Design review of the part shown in the three views and the two pictorial views. Dimensions are in mm from the part's minimum x, y and z. A direction names the side the tool comes from. Round coordinates to 2 decimals unless told otherwise and drop trailing zeros. Order: outer loops, then holes, each group sorted by start corner. A loop starts at its lowest first (then second) coordinate and runs counter-clockwise, first axis right, second up.
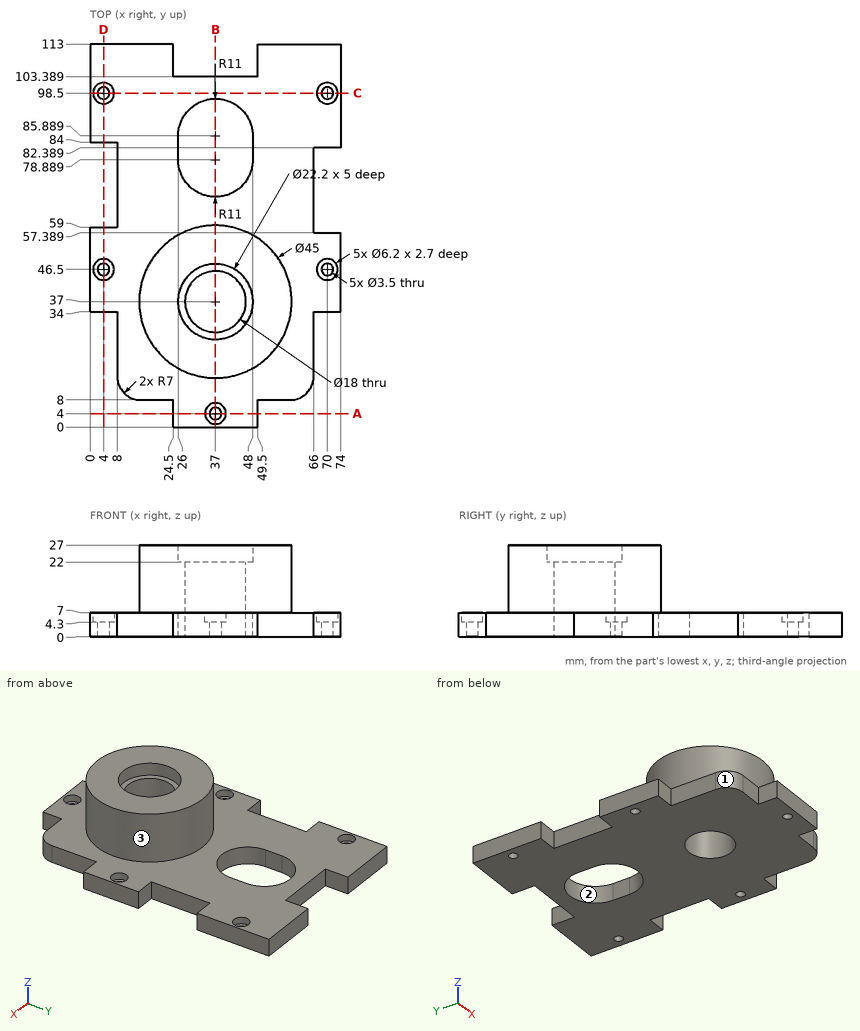
(1) For the marked faces 1, 2 and 3, list the 3-axis set-ups (+Z, -Z, +X, -X, +Y, -Y) from which the entire face can be reached by the end or side of a thin tool; tool diameter is ignored.
Data:
face 1: +Z, -Z, -X, -Y
face 2: +Z, -Z
face 3: +Z
(2) Consider section C-C (y = 98.5). Write out the cut boundary in (x, z).
Data:
outline: (0, 0) - (2.25, 0) - (2.25, 4.3) - (0.9, 4.3) - (0.9, 7) - (0, 7) - close; (5.75, 0) - (68.25, 0) - (68.25, 4.3) - (66.9, 4.3) - (66.9, 7) - (7.1, 7) - (7.1, 4.3) - (5.75, 4.3) - close; (71.75, 0) - (74, 0) - (74, 7) - (73.1, 7) - (73.1, 4.3) - (71.75, 4.3) - close
(3) Consider section B-B (x = 37). Write out the cut boundary in (y, z), and give its area (3 significant figures).
Data:
outline: (0, 0) - (2.25, 0) - (2.25, 4.3) - (0.9, 4.3) - (0.9, 7) - (0, 7) - close; (5.75, 0) - (28, 0) - (28, 22) - (25.9, 22) - (25.9, 27) - (14.5, 27) - (14.5, 7) - (7.1, 7) - (7.1, 4.3) - (5.75, 4.3) - close; (46, 0) - (67.89, 0) - (67.89, 7) - (59.5, 7) - (59.5, 27) - (48.1, 27) - (48.1, 22) - (46, 22) - close; (96.89, 0) - (103.39, 0) - (103.39, 7) - (96.89, 7) - close
area: 882 mm2
(4) To check wall thickness, follow probe 1 along Y at (x, z) = (70, 1.45); probe 2 along Y at (x, z) = (70, 5); probe 3 along Y at (x, z) = (37, 18). State the ranges of each line that lie inside material, in increasing order.
Data:
probe 1: y = 34 to 44.75, 48.25 to 57.39, 82.39 to 96.75, 100.25 to 113
probe 2: y = 34 to 43.4, 49.6 to 57.39, 82.39 to 95.4, 101.6 to 113
probe 3: y = 14.5 to 28, 46 to 59.5
(5) Consider section A-A (y = 4). Write out the cut boundary in (x, z).
Data:
outline: (24.5, 0) - (35.25, 0) - (35.25, 4.3) - (33.9, 4.3) - (33.9, 7) - (24.5, 7) - close; (38.75, 0) - (49.5, 0) - (49.5, 7) - (40.1, 7) - (40.1, 4.3) - (38.75, 4.3) - close
(6) Consider section D-D (x = 4). Write out the cut boundary in (y, z).
Data:
outline: (34, 0) - (44.75, 0) - (44.75, 4.3) - (43.4, 4.3) - (43.4, 7) - (34, 7) - close; (48.25, 0) - (59, 0) - (59, 7) - (49.6, 7) - (49.6, 4.3) - (48.25, 4.3) - close; (84, 0) - (96.75, 0) - (96.75, 4.3) - (95.4, 4.3) - (95.4, 7) - (84, 7) - close; (100.25, 0) - (113, 0) - (113, 7) - (101.6, 7) - (101.6, 4.3) - (100.25, 4.3) - close
(7) Insertion check: pin 1 (3 mm diameter, centred on x = 71.5, y = 99.5, fed in from +Z); pin 2 (3.5 mm diameter, centred on y = 23, z = 3, fed in from -X); pin 3 (6 mm diameter, centred on y = 87, z = 11.5, fed in from -X) (3 decimals); pin 4 (7.5 mm diameter, centred on x = 55, z = 5, fed in from -Y). Each pin has a flat end and moves straight along its axis. Give the tip position at first contact, or say it passes through.
Data:
pin 1: stops at z = 7
pin 2: stops at x = 8
pin 3: passes through
pin 4: stops at y = 8
